Can you work these out from the model? Positions are in its coordinate system, mm. A direction names the side the tool comes from. Coordinates: 2 decimals unless noted, no trailing zeros. Loops run counter-clockwise (first coordinate to the right, second up) from the corner with the lowest first, then second, coordinate; pieces in that order, holes last.
```python
from build123d import *

# Parameters (mm, degrees)
SKETCH1_R                = 13
SKETCH1_W                = 48
SKETCH1_H                = 8
BOSS_EXTRUDE1_DEPTH      = 13.5
SKETCH2_R                = 11.15
CUT_EXTRUDE1_DEPTH       = 5
SKETCH2_3_R              = 5.075
CUT_EXTRUDE2_DEPTH       = 41.360872141
SKETCH3_R                = 6.1
CUT_EXTRUDE3_DEPTH       = 10
CUT_EXTRUDE4_DEPTH       = 41.360872141
SKETCH5_R                = 3.25
CUT_EXTRUDE5_DEPTH       = 33.897568299
M3_CLEARANCE_HOLE1_D     = 3.4
CUT_EXTRUDE6_DEPTH       = 5
CIRPATTERN1_COUNT        = 4
BOSS_EXTRUDE2_START      = -13.5
BOSS_EXTRUDE2_DEPTH      = 27
M3_CLEARANCE_HOLE2_D     = 3.4
M3_CLEARANCE_HOLE2_DEPTH = 12
M3_CLEARANCE_HOLE2_TIP   = 1.021463052
CUT_EXTRUDE7_START       = -5
SKETCH12_R               = 1.7
CUT_EXTRUDE7_DEPTH       = 3
CUT_EXTRUDE8_DEPTH       = 49.592694924


with BuildPart() as part:
    # Sketch1 → Boss-Extrude1 (new, symmetric)
    with BuildSketch(Plane.XY):
        with BuildLine():
            ThreePointArc((-8.306623863, 10), (-13, 0), (-8.306623863, -10))
            Line((-8.306623863, -10), (8.306623863, -10))
            ThreePointArc((8.306623863, -10), (11.768307232, -5.523309234), (13, 0))
            ThreePointArc((13, 0), (11.768307232, 5.523309234), (8.306623863, 10))
            Line((8.306623863, 10), (-8.306623863, 10))
        make_face()
        with BuildLine():
            ThreePointArc((8.306623863, 10), (0, 13), (-8.306623863, 10))
            Line((-8.306623863, 10), (8.306623863, 10))
        make_face()
        with BuildLine():
            ThreePointArc((13, 0), (11.768307232, -5.523309234), (8.306623863, -10))
            Line((8.306623863, -10), (24, -10))
            Line((24, -10), (24, 10))
            Line((24, 10), (8.306623863, 10))
            ThreePointArc((8.306623863, 10), (11.768307232, 5.523309234), (13, 0))
        make_face()
        with BuildLine():
            Line((8.306623863, -10), (-8.306623863, -10))
            ThreePointArc((-8.306623863, -10), (0, -13), (8.306623863, -10))
        make_face()
        with BuildLine():
            Line((-24, 10), (-24, -10))
            Line((-24, -10), (-8.306623863, -10))
            ThreePointArc((-8.306623863, -10), (-13, 0), (-8.306623863, 10))
            Line((-8.306623863, 10), (-24, 10))
        make_face()
        Circle(SKETCH1_R)
        with Locations((0, -14)):
            Rectangle(SKETCH1_W, SKETCH1_H)
    extrude(amount=BOSS_EXTRUDE1_DEPTH, both=True)

    # Sketch2 → Cut-Extrude1 (cut)
    with BuildSketch(Plane(origin=(0, 0, -13.5), x_dir=(-1, 0, 0), z_dir=(0, 0, -1))):
        Circle(SKETCH2_R)
    extrude(amount=-CUT_EXTRUDE1_DEPTH, mode=Mode.SUBTRACT)

    # Sketch2<3> → Cut-Extrude2 (cut, through all)
    with BuildSketch(Plane(origin=(0, 0, -13.5), x_dir=(-1, 0, 0), z_dir=(0, 0, -1))):
        Circle(SKETCH2_3_R)
    extrude(amount=-CUT_EXTRUDE2_DEPTH, mode=Mode.SUBTRACT)

    # Sketch3 → Cut-Extrude3 (cut, symmetric)
    with BuildSketch(Plane.XY):
        with Locations((-14.26606865, -8)):
            Circle(SKETCH3_R)
        with BuildLine():
            ThreePointArc((-14.26606865, -14.1), (-20.36606865, -8), (-14.26606865, -1.9))
            Line((-14.26606865, -1.9), (-24, -1.9))
            Line((-24, -1.9), (-24, -14.1))
            Line((-24, -14.1), (-14.26606865, -14.1))
        make_face()
    cut_extrude3 = extrude(amount=CUT_EXTRUDE3_DEPTH, both=True, mode=Mode.SUBTRACT)

    # Sketch4 → Cut-Extrude4 (cut, through all)
    with BuildSketch(Plane(origin=(0, 0, -13.5), x_dir=(-1, 0, 0), z_dir=(0, 0, -1))):
        with BuildLine():
            Line((18, 2.1), (24, 2.1))
            Line((24, 2.1), (24, 10))
            Line((24, 10), (8.306623863, 10))
            ThreePointArc((8.306623863, 10), (10.1107181, 8.171497996), (11.520065039, 6.023960615))
            ThreePointArc((11.520065039, 6.023960615), (14.212288818, 3.157449424), (18, 2.1))
        make_face()
    cut_extrude4 = extrude(amount=-CUT_EXTRUDE4_DEPTH, mode=Mode.SUBTRACT)

    # Sketch5 → Cut-Extrude5 (cut, symmetric)
    with BuildSketch(Plane.XY):
        with Locations((-14.26606865, -8)):
            Circle(SKETCH5_R)
    cut_extrude5 = extrude(amount=CUT_EXTRUDE5_DEPTH, both=True, mode=Mode.SUBTRACT)

    # Mirror1: Cut-Extrude3, Cut-Extrude4, Cut-Extrude5 across plane
    add(cut_extrude3.mirror(Plane(origin=(0, 0, 0), x_dir=(0, 0, 1), z_dir=(1, 0, 0))), mode=Mode.SUBTRACT)
    add(cut_extrude4.mirror(Plane(origin=(0, 0, 0), x_dir=(0, 0, 1), z_dir=(1, 0, 0))), mode=Mode.SUBTRACT)
    add(cut_extrude5.mirror(Plane(origin=(0, 0, 0), x_dir=(0, 0, 1), z_dir=(1, 0, 0))), mode=Mode.SUBTRACT)

    # M3 Clearance Hole1 (through all)
    with Locations(Plane(origin=(0, 0, -8.5), x_dir=(-1, 0, 0), z_dir=(0, 0, -1))):
        with Locations((0, -8), (-8, 0), (0, 8), (8, 0)):
            Hole(M3_CLEARANCE_HOLE1_D / 2)

    # Sketch8 → Cut-Extrude6 (cut)
    with BuildSketch(Plane.XY.offset(13.5)):
        Polygon((-10.8, -1.616580754), (-8, -3.233161507), (-5.2, -1.616580754), (-5.2, 1.616580754), (-8, 3.233161507), (-10.8, 1.616580754), align=None)
    cut_extrude6 = extrude(amount=-CUT_EXTRUDE6_DEPTH, mode=Mode.SUBTRACT)

    # CirPattern1: Cut-Extrude6 ×4 about axis
    cirpattern1_axis = Axis((0, 0, 0), (0, 0, 1))
    for i in range(1, CIRPATTERN1_COUNT):
        add(cut_extrude6.rotate(cirpattern1_axis, i * 360 / CIRPATTERN1_COUNT), mode=Mode.SUBTRACT)

    # Sketch9 → Boss-Extrude2 (add)
    with BuildSketch(Plane.XY.offset(BOSS_EXTRUDE2_START)):
        Polygon((12, -32.5), (24, -32.5), (24, -18), (-24, -18), (-24, -32.5), (-12, -32.5), (-13, -27.5), (13, -27.5), align=None)
    extrude(amount=BOSS_EXTRUDE2_DEPTH)

    # M3 Clearance Hole2
    with Locations(Plane(origin=(0, -32.5, 0), x_dir=(-1, 0, 0), z_dir=(0, -1, 0))):
        with Locations((-18.5, 0), (18.5, 0)):
            Hole(M3_CLEARANCE_HOLE2_D / 2, depth=M3_CLEARANCE_HOLE2_DEPTH)
            with Locations((0, 0, -(M3_CLEARANCE_HOLE2_DEPTH + M3_CLEARANCE_HOLE2_TIP / 2))):  # 118° drill point
                Cone(0, M3_CLEARANCE_HOLE2_D / 2, M3_CLEARANCE_HOLE2_TIP, mode=Mode.SUBTRACT)

    # Sketch12 → Cut-Extrude7 (cut)
    # profile 1 of 4: a face of its own
    with BuildSketch(Plane.XZ.offset(32.5).offset(CUT_EXTRUDE7_START)):
        Polygon((20.116580754, -2.8), (21.733161507, 0), (20.116580754, 2.8), (16.883419246, 2.8), (15.266838493, 0), (16.883419246, -2.8), align=None)
    # profile 2 of 4: a face of its own
    with BuildSketch(Plane.XZ.offset(32.5).offset(CUT_EXTRUDE7_START)):
        Polygon((24, -2.8), (20.116580754, -2.8), (21.733161507, 0), (20.116580754, 2.8), (24, 2.8), align=None)
    # profile 3 of 4: a face of its own
    with BuildSketch(Plane.XZ.offset(32.5).offset(CUT_EXTRUDE7_START)):
        Polygon((-15.266838493, 0), (-16.883419246, 2.8), (-20.116580754, 2.8), (-21.733161507, 0), (-20.116580754, -2.8), (-16.883419246, -2.8), align=None)
        with Locations(Location((-18.5, 0, 0), (0, 0, 270))):
            Circle(SKETCH12_R, mode=Mode.SUBTRACT)
    # profile 4 of 4: a face of its own
    with BuildSketch(Plane.XZ.offset(32.5).offset(CUT_EXTRUDE7_START)):
        Polygon((-21.733161507, 0), (-20.116580754, 2.8), (-24, 2.8), (-24, -2.8), (-20.116580754, -2.8), align=None)
    extrude(amount=CUT_EXTRUDE7_DEPTH, mode=Mode.SUBTRACT)

    # Sketch13 → Cut-Extrude8 (cut, through all)
    with BuildSketch(Plane.XY.offset(13.5)):
        Polygon((-12.098058068, -32.519611614), (12.098058068, -32.519611614), (13.12198039, -27.4), (-13.12198039, -27.4), align=None)
    extrude(amount=-CUT_EXTRUDE8_DEPTH, mode=Mode.SUBTRACT)


solid = part.part
```
Item 1: Suppose I cut it at C-C, the plane z = 5.5. Please give me the cut outline in (x, y) (3 decimals).
Results are:
outline: (-24, -32.5) - (-12.102, -32.5) - (-13.122, -27.4) - (13.122, -27.4) - (12.102, -32.5) - (24, -32.5) - (24, -14.1) - (14.266, -14.1) arc R6.1 cw to (14.266, -1.9) - (24, -1.9) - (24, 2.1) - (18, 2.1) arc R7.312 cw to (11.52, 6.024) arc R13 ccw to (-11.52, 6.024) arc R7.312 cw to (-18, 2.1) - (-24, 2.1) - (-24, -1.9) - (-14.266, -1.9) arc R6.1 cw to (-14.266, -14.1) - (-24, -14.1) - close; hole circle Ø3.4 at (-8, 0); hole circle Ø10.15 at (0, 0); hole circle Ø3.4 at (0, -8); hole circle Ø3.4 at (0, 8); hole circle Ø3.4 at (8, 0)
Item 2: Suppose I cut it at B-B, the plane x = -0.5. Please give me the cut outline in (y, z), plus the area to 3 significant figures.
Results are:
outline: (-27.4, -13.5) - (-11.14, -13.5) - (-11.14, -8.5) - (-9.62, -8.5) - (-9.62, 8.5) - (-10.8, 8.5) - (-10.8, 13.5) - (-27.4, 13.5) - close; (-6.38, -8.5) - (-5.05, -8.5) - (-5.05, 13.5) - (-5.2, 13.5) - (-5.2, 8.5) - (-6.38, 8.5) - close; (5.05, -8.5) - (6.38, -8.5) - (6.38, 8.5) - (5.2, 8.5) - (5.2, 13.5) - (5.05, 13.5) - close; (9.62, -8.5) - (11.14, -8.5) - (11.14, -13.5) - (12.99, -13.5) - (12.99, 13.5) - (10.8, 13.5) - (10.8, 8.5) - (9.62, 8.5) - close
area: 590 mm2
Item 3: I'm going to push flat-ended pins straight in: P1, Ø1.5, axis at x = -5, z = -11, coming from the +Y side; P2, Ø1, axis at y = -12.5, z = 3, coming from the -X side; P3, Ø2, axis at y = -7, z = -1, coming from the +X side; P4, Ø6.5, axis at x = -1, y = -1, coming from the -Z side. Where does each tip first touch, or does it pass through?
Results are:
P1: stops at y = 12.29
P2: stops at x = -10.77
P3: stops at x = 8.5
P4: passes through
Item 4: We'd pull the mould along X, two halves only. Please class faces 1 (the face through (-10.8, 0, 11)), 2 (the face through (16.086, -28.979, 1.42)), 3 (the face through (18, -8, -10)): +X half, -X half, draft (parallel to the pull), parting line (faces both ways), or undercut.
Results are:
face 1: undercut
face 2: +X half
face 3: draft
Item 5: I need wall thicknesses on line 1 along Y through (x, z) = (21, 0.25); line 2 along X through (y, z) = (0, -10.8); line 3 along Z through (x, y) = (-15, -12). Which ranges of each line are inside material? Lowest first, please.
Results are:
line 1: y = -32.5 to -30.5, -27.5 to -14.1, -1.9 to 2.1
line 2: x = -24 to -11.15, 11.15 to 24
line 3: z = -13.5 to -10, 10 to 13.5
Item 6: Suppose I cut it at D-D, the plane y = 7. Please give me the cut outline in (x, z), plus the area to 3 significant figures.
Results are:
outline: (-10.95, -13.5) - (-8.68, -13.5) - (-8.68, -8.5) - (-1.37, -8.5) - (-1.37, 8.5) - (-2.66, 8.5) - (-2.66, 13.5) - (-10.95, 13.5) - close; (1.37, -8.5) - (8.68, -8.5) - (8.68, -13.5) - (10.95, -13.5) - (10.95, 13.5) - (2.66, 13.5) - (2.66, 8.5) - (1.37, 8.5) - close
area: 431 mm2
Item 7: Suppose I cut it at A-A, the plane y = 0. Please give me the cut outline in (x, z) (3 decimals).
Results are:
outline: (-24, -13.5) - (-11.15, -13.5) - (-11.15, -8.5) - (-9.7, -8.5) - (-9.7, 8.5) - (-10.8, 8.5) - (-10.8, 13.5) - (-24, 13.5) - close; (-6.3, -8.5) - (-5.075, -8.5) - (-5.075, 13.5) - (-5.2, 13.5) - (-5.2, 8.5) - (-6.3, 8.5) - close; (5.075, -8.5) - (6.3, -8.5) - (6.3, 8.5) - (5.2, 8.5) - (5.2, 13.5) - (5.075, 13.5) - close; (9.7, -8.5) - (11.15, -8.5) - (11.15, -13.5) - (24, -13.5) - (24, 13.5) - (10.8, 13.5) - (10.8, 8.5) - (9.7, 8.5) - close
Item 8: On a 3-axis mill with a long thin cutter (end or side, diameter ignored), from which of +Z, -Z, +X, -X, +Y, -Y can I reach the whole of each face in a straight line? I mean faces 4 (the face through (-2.414, 9.42, 11.035)), 5 (the face through (-16.086, -28.979, -1.42)), 6 (the face through (0, -14, 13.5)), 7 (the face through (16.6, -32.5, -0.2)), 8 (the face through (-12.62, -29.91, 0.19)). Say none if no direction works.
Results are:
face 4: +Z
face 5: -X
face 6: +Z, +X, -X, +Y, -Y
face 7: +Z, -Z, +X, -X, -Y
face 8: +Z, -Z
